```python
from build123d import *

# Parameters (mm, degrees)
ESBO_O4_W                = 84
ESBO_O4_H                = 50
RESSALTO_EXTRUS_O2_DEPTH = 3
CORTE_EXTRUS_O2_REACH    = 50.969
ESBO_O5_W                = 12
ESBO_O5_H                = 3
CORTE_EXTRUS_O4_REACH    = 50.969
ESBO_O6_W                = 3
ESBO_O6_H                = 10
CORTE_EXTRUS_O5_REACH    = 50.969
ESBO_O8_R                = 2.5
ESBO_O8_W                = 15
ESBO_O8_H                = 15
ESBO_O11_W               = 3
ESBO_O11_H               = 10
RESSALTO_EXTRUS_O4_DEPTH = 6


with BuildPart() as part:
    # Esboço4 → Ressalto-extrusão2 (new body)
    with BuildSketch(Plane.XY):
        Rectangle(ESBO_O4_W, ESBO_O4_H)
    extrude(amount=RESSALTO_EXTRUS_O2_DEPTH)

    # Esboço5 → Corte-extrusão2 (cut, up to next)
    with BuildSketch(Plane.XY.offset(3), mode=Mode.PRIVATE) as corte_extrus_o2_sk1:
        with Locations((24, 23.5)):
            Rectangle(ESBO_O5_W, ESBO_O5_H)
    corte_extrus_o2_tool1 = extrude(corte_extrus_o2_sk1.sketch, amount=-CORTE_EXTRUS_O2_REACH, mode=Mode.PRIVATE) & part.part
    # Esboço5 → Corte-extrusão2 (cut, up to next)
    with BuildSketch(Plane.XY.offset(3), mode=Mode.PRIVATE) as corte_extrus_o2_sk2:
        with Locations((-24, 23.5)):
            Rectangle(ESBO_O5_W, ESBO_O5_H)
    corte_extrus_o2_tool2 = extrude(corte_extrus_o2_sk2.sketch, amount=-CORTE_EXTRUS_O2_REACH, mode=Mode.PRIVATE) & part.part
    # Esboço5 → Corte-extrusão2 (cut, up to next)
    with BuildSketch(Plane.XY.offset(3), mode=Mode.PRIVATE) as corte_extrus_o2_sk3:
        with Locations((0, 23.5)):
            Rectangle(ESBO_O5_W, ESBO_O5_H)
    corte_extrus_o2_tool3 = extrude(corte_extrus_o2_sk3.sketch, amount=-CORTE_EXTRUS_O2_REACH, mode=Mode.PRIVATE) & part.part
    # Esboço5 → Corte-extrusão2 (cut, up to next)
    with BuildSketch(Plane.XY.offset(3), mode=Mode.PRIVATE) as corte_extrus_o2_sk4:
        with Locations((0, -23.5)):
            Rectangle(ESBO_O5_W, ESBO_O5_H)
    corte_extrus_o2_tool4 = extrude(corte_extrus_o2_sk4.sketch, amount=-CORTE_EXTRUS_O2_REACH, mode=Mode.PRIVATE) & part.part
    # Esboço5 → Corte-extrusão2 (cut, up to next)
    with BuildSketch(Plane.XY.offset(3), mode=Mode.PRIVATE) as corte_extrus_o2_sk5:
        with Locations((-24, -23.5)):
            Rectangle(ESBO_O5_W, ESBO_O5_H)
    corte_extrus_o2_tool5 = extrude(corte_extrus_o2_sk5.sketch, amount=-CORTE_EXTRUS_O2_REACH, mode=Mode.PRIVATE) & part.part
    # Esboço5 → Corte-extrusão2 (cut, up to next)
    with BuildSketch(Plane.XY.offset(3), mode=Mode.PRIVATE) as corte_extrus_o2_sk6:
        with Locations((24, -23.5)):
            Rectangle(ESBO_O5_W, ESBO_O5_H)
    corte_extrus_o2_tool6 = extrude(corte_extrus_o2_sk6.sketch, amount=-CORTE_EXTRUS_O2_REACH, mode=Mode.PRIVATE) & part.part
    add(corte_extrus_o2_tool1.solids().sort_by_distance((24, 23.5, 3))[0], mode=Mode.SUBTRACT)
    add(corte_extrus_o2_tool2.solids().sort_by_distance((-24, 23.5, 3))[0], mode=Mode.SUBTRACT)
    add(corte_extrus_o2_tool3.solids().sort_by_distance((0, 23.5, 3))[0], mode=Mode.SUBTRACT)
    add(corte_extrus_o2_tool4.solids().sort_by_distance((0, -23.5, 3))[0], mode=Mode.SUBTRACT)
    add(corte_extrus_o2_tool5.solids().sort_by_distance((-24, -23.5, 3))[0], mode=Mode.SUBTRACT)
    add(corte_extrus_o2_tool6.solids().sort_by_distance((24, -23.5, 3))[0], mode=Mode.SUBTRACT)

    # Esboço6 → Corte-extrusão4 (cut, up to next)
    with BuildSketch(Plane.XY, mode=Mode.PRIVATE) as corte_extrus_o4_sk1:
        with Locations((40.5, 10)):
            Rectangle(ESBO_O6_W, ESBO_O6_H)
    corte_extrus_o4_tool1 = extrude(corte_extrus_o4_sk1.sketch, amount=CORTE_EXTRUS_O4_REACH, mode=Mode.PRIVATE) & part.part
    # Esboço6 → Corte-extrusão4 (cut, up to next)
    with BuildSketch(Plane.XY, mode=Mode.PRIVATE) as corte_extrus_o4_sk2:
        with Locations((-40.5, 10)):
            Rectangle(ESBO_O6_W, ESBO_O6_H)
    corte_extrus_o4_tool2 = extrude(corte_extrus_o4_sk2.sketch, amount=CORTE_EXTRUS_O4_REACH, mode=Mode.PRIVATE) & part.part
    # Esboço6 → Corte-extrusão4 (cut, up to next)
    with BuildSketch(Plane.XY, mode=Mode.PRIVATE) as corte_extrus_o4_sk3:
        with Locations((-40.5, -10)):
            Rectangle(ESBO_O6_W, ESBO_O6_H)
    corte_extrus_o4_tool3 = extrude(corte_extrus_o4_sk3.sketch, amount=CORTE_EXTRUS_O4_REACH, mode=Mode.PRIVATE) & part.part
    # Esboço6 → Corte-extrusão4 (cut, up to next)
    with BuildSketch(Plane.XY, mode=Mode.PRIVATE) as corte_extrus_o4_sk4:
        with Locations((40.5, -10)):
            Rectangle(ESBO_O6_W, ESBO_O6_H)
    corte_extrus_o4_tool4 = extrude(corte_extrus_o4_sk4.sketch, amount=CORTE_EXTRUS_O4_REACH, mode=Mode.PRIVATE) & part.part
    add(corte_extrus_o4_tool1.solids().sort_by_distance((40.5, 10, 0))[0], mode=Mode.SUBTRACT)
    add(corte_extrus_o4_tool2.solids().sort_by_distance((-40.5, 10, 0))[0], mode=Mode.SUBTRACT)
    add(corte_extrus_o4_tool3.solids().sort_by_distance((-40.5, -10, 0))[0], mode=Mode.SUBTRACT)
    add(corte_extrus_o4_tool4.solids().sort_by_distance((40.5, -10, 0))[0], mode=Mode.SUBTRACT)

    # Esboço8 → Corte-extrusão5 (cut, up to next)
    with BuildSketch(Plane(origin=(0, 0, 0), x_dir=(-1, 0, 0), z_dir=(0, 0, -1)), mode=Mode.PRIVATE) as corte_extrus_o5_sk1:
        with Locations((13.99726894, 13)):
            Circle(ESBO_O8_R)
    corte_extrus_o5_tool1 = extrude(corte_extrus_o5_sk1.sketch, amount=-CORTE_EXTRUS_O5_REACH, mode=Mode.PRIVATE) & part.part
    # Esboço8 → Corte-extrusão5 (cut, up to next)
    with BuildSketch(Plane(origin=(0, 0, 0), x_dir=(-1, 0, 0), z_dir=(0, 0, -1)), mode=Mode.PRIVATE) as corte_extrus_o5_sk2:
        with Locations((13.657630315, -7)):
            Rectangle(ESBO_O8_W, ESBO_O8_H)
    corte_extrus_o5_tool2 = extrude(corte_extrus_o5_sk2.sketch, amount=-CORTE_EXTRUS_O5_REACH, mode=Mode.PRIVATE) & part.part
    add(corte_extrus_o5_tool1.solids().sort_by_distance((-13.997269, 13, 0))[0], mode=Mode.SUBTRACT)
    add(corte_extrus_o5_tool2.solids().sort_by_distance((-13.65763, -7, 0))[0], mode=Mode.SUBTRACT)

    # Esboço11 → Ressalto-extrusão4 (add)
    with BuildSketch(Plane.ZY.offset(42)):
        with Locations((1.5, 0)):
            Rectangle(ESBO_O11_W, ESBO_O11_H)
        with Locations((1.5, 20)):
            Rectangle(ESBO_O11_W, ESBO_O11_H)
    extrude(amount=RESSALTO_EXTRUS_O4_DEPTH)


solid = part.part
```
Geometry: final body of the model. Coordinates: model frame, mm. A direction names the side the tool comes from. Round coordinates to 2 decimals unless told otherwise and drop trailing zeros. Write each loop counter-clockwise with the first axis right and the second up, starting at its lowest first coordinate (ties: lowest second). Pieces come first, ordered by that corner, then holes.
Item 1: Section query B-B (y = 13). Return loops of the section in (x, z), plus the area to 3 significant figures.
Item 2: Pin query (flat end, axial travel): P1, Ø0.9, axis at x = -24.5, z = 1, coming from the -Y side; P2, Ø1.5, axis at y = -22, z = 1, coming from the -X side; P3, Ø1.5, axis at x = -1, z = 1, coming from the +Y side. Return the tip coordinate at first contact, or that it passes through.
Item 3: Section query D-D (y = -17.5). Return loops of the section in (x, z).
Item 4: Mould query, pull axis Y, two halves, no side actions, for faces 5 (the face through (-30, 23, 2)), 6 (the face through (24, -22, 2)), 7 (the face through (40, 15, 1)). Classes: +Y half, -Y half, draft (parallel to the pull), parting line (faces both ways), or undercut.
Item 5: Set-up query: faces 1 (the face through (24, 22, 2)), 2 (the face through (40, -15, 1)), 3 (the face through (-14, -14.5, 1)), 4 (the face through (-18, -24, 2)). Return all of +Z, -Z, +X, -X, +Y, -Y with unobstructed straight access to the full face (end or side cutting, diameter ignored); none if empty.
Item 6: Section query C-C (z = 0.95). Give the number of separate pieces and of enclosed holes in the cut face, plus the area to 3 significant figures.
Item 7: Section query A-A (y = -10). Return loops of the section in (x, z).
Item 8: Material intervals for L1, parallel to Y at x = -43.5, z = 1.95; L2, parallel to X at y = -11, z = 0.9; L3, parallel to X at y = -1, z = 1.85, sorted ascending.
Completed:
1. outline: (-39, 0) - (-16.5, 0) - (-16.5, 3) - (-39, 3) - close; (-11.5, 0) - (39, 0) - (39, 3) - (-11.5, 3) - close
1. area: 219 mm2
2. P1: stops at y = -22
2. P2: stops at x = -42
2. P3: stops at y = 22
3. outline: (-42, 0) - (42, 0) - (42, 3) - (-42, 3) - close
4. face 5: draft
4. face 6: -Y half
4. face 7: undercut
5. face 1: +Z, -Z, +Y
5. face 2: +Z, -Z, +X
5. face 3: +Z, -Z
5. face 4: +Z, -Z, -Y
6. separate pieces: 1
6. enclosed holes: 2
6. area: 3,740 mm2
7. outline: (-39, 0) - (-21.16, 0) - (-21.16, 3) - (-39, 3) - close; (-6.16, 0) - (39, 0) - (39, 3) - (-6.16, 3) - close
8. L1: y = -5 to 5, 15 to 25
8. L2: x = -39 to -21.16, -6.16 to 39
8. L3: x = -48 to -21.16, -6.16 to 42
